Source: CAD feature listing. Evaluate the final solid. Frame: model axes, mm. A direction names the side the tool comes from. Round coordinates to 2 decimals unless told otherwise and drop trailing zeros. Loops run counter-clockwise (first coordinate to the right, second up) from the corner with the lowest first, then second, coordinate; pieces in that order, holes last. Notation, with made-up numbers: M 66.5,30.5 L 89.5,30.5 A13 cw 89.5,44.5 Z; hole C -25,0 d10. An arc over 180 degrees is marked long. Answer as CSV lines item,"result". Start each with the question number.
Autodesk Fusion 360 part; units mm, degrees
sketch "Sketch1" plane through (0, 0, 0) normal (0, 0, 1) x (1, 0, 0)
  line L0 (9, 9) -> (-9, 9) construction
  line L1 (-9, 9) -> (-9, -9) construction
  line L2 (-9, -9) -> (9, -9) construction
  line L3 (9, -9) -> (9, 9) construction
  line L4 (9, 9) -> (-9, -9) construction
  line L5 (-9, 9) -> (9, -9) construction
  line L6 (-6.4, 8) -> (6.4, 8)
  line L7 (6.4, 8) -> (6.4, -5.4)
  line L8 (6.4, -5.4) -> (-6.4, -5.4)
  line L9 (-6.4, -5.4) -> (-6.4, 8)
  circle A0 centre (0, 0) radius 3.5
  line L10 (2.4, -0.6) -> (-2.4, -0.6)
  line L11 (-2.4, -0.6) -> (-2.4, 0.6)
  line L12 (-2.4, 0.6) -> (2.4, 0.6)
  line L13 (2.4, 0.6) -> (2.4, -0.6)
  line L14 (2.4, -0.6) -> (-2.4, 0.6) construction
  line L15 (-2.4, -0.6) -> (2.4, 0.6) construction
  line L16 (0.6, -2.4) -> (-0.6, -2.4)
  line L17 (-0.6, -2.4) -> (-0.6, 2.4)
  line L18 (-0.6, 2.4) -> (0.6, 2.4)
  line L19 (0.6, 2.4) -> (0.6, -2.4)
  line L20 (0.6, -2.4) -> (-0.6, 2.4) construction
  line L21 (-0.6, -2.4) -> (0.6, 2.4) construction
  line L22 (-0.6, 2.4) -> (-2.5475, 2.4)
  line L23 (0.6, 2.4) -> (2.5475, 2.4)
  line L24 (-0.6, -2.4) -> (-2.5475, -2.4)
  line L25 (0.6, -2.4) -> (2.5475, -2.4)
  dimension "d1" = 18
  dimension "d2" = 18
  dimension "d3" = 3.6
  dimension "d4" = 1
  dimension "d5" = 2.6
  dimension "d6" = 2.6
  dimension "d7" = 7
  dimension "d8" = 4.8
  dimension "d9" = 1.2
  dimension "d10" = 1.2
  dimension "d11" = 4.8
extrude "Extrude1" add sketch "Sketch1" along normal blind 0.6 contours L6 L7 L8 L9 | A0 L10 L12 L13 L19 L23 L25 | A0 L18 L22 L23 | A0 L16 L24 L25 | A0 L10 L11 L12 L17 L22 L24 | L12 L17 L18 L19 | L10 L16 L17 L19 | L10 L12 L17 L19 | L10 L12 L13 L19 | L10 L11 L12 L17
extrude "Extrude2" add sketch "Sketch1" along normal blind 4 contours A0 L10 L12 L13 L19 L23 L25 | A0 L10 L11 L12 L17 L22 L24
fillet "Fillet1" radius 1 6 edges at (-1.5738, -2.4, 0.6) (-3.5, 0, 0.6) (1.5738, -2.4, 0.6) (3.5, 0, 0.6) (1.5738, 2.4, 0.6) (-1.5738, 2.4, 0.6)
fillet "Fillet1" radius 0.5 4 edges at (6.4, 8, 0.3) (-6.4, 8, 0.3) (6.4, -5.4, 0.3) (-6.4, -5.4, 0.3)
chamfer "Chamfer1" distance 0.4 angle 45 20 edges at (-6.2536, 7.8536, 0) (0, 8, 0) (6.2536, 7.8536, 0) (6.4, 1.3, 0) (6.2536, -5.2536, 0) (0, -5.4, 0) (-6.2536, -5.2536, 0) (-6.4, 1.3, 0) (-0.6, 1.5, 4) (-1.5, 0.6, 4) (-2.4, 0, 4) (-1.5, -0.6, 4) (-0.6, -1.5, 4) (0.6, -1.5, 4) (1.5, -0.6, 4) (2.4, 0, 4) (1.5, 0.6, 4) (0.6, 1.5, 4) (3.5, 0, 4) (-3.5, 0, 4)
1) Section C-C, the plane y = 3.75. Return loops of the section in (x, z).
2) Ray query, line 1 along X through (y, z) = (0, 2.9); line 2 along Y through (x, z) = (0.75, 3.5); line 3 along Z through (x, y) = (-2.25, -3.5). Return the intervals inside material, ascending.
3) Section D-D, the plane x = 5.5. Return loops of the section in (y, z), and give its area (3 significant figures).
4) Contact query for flat-ended pins moving along their axis: pin 1 Ø0.8 at (y, z) = (-2, 2.5) entering from -X; pin 2 Ø2 at (x, z) = (1.5, 2.5) entering from -Y (3 decimals); pin 3 Ø2 at (x, z) = (1.5, 3) entering from +Y. Output: stop coordinate, or through.
5) Access query for faces 1 (the flat face through (-2.4, 0, 2)), 2 (the flat face through (-0.6, 2, 2)), 3 (the flat face through (2, 2.4, 3)). Directions: +Z, -Z, +X, -X, +Y, -Y. A direction counts if a zero-diameter tool reaches every point of the face in a straight line with its end or side. Return the directions, or none.
6) Mould query, pull axis X, two halves, no side actions, for faces 4 (the flat face through (0, 1, 0)), 5 (the conical face through (3.21, 0.04, 3.89)), 6 (the flat face through (1, 0.6, 2)). Classes: pulls with the +X half, pulls with the -X half, needs draft (parallel to the pull), parting line crosses it, or undercut.
7) Section A-A, the plane x = -1.5. Return loops of the section in (y, z), and give its area (3 significant figures).
8) Section B-B, the plane z = 2.35. Return loops of the section in (x, y), and give its area (3 significant figures).
Findings below:
1,outline,"M -6.4,0.4 L -6,0 L 6,0 L 6.4,0.4 L 6.4,0.6 L -6.4,0.6 Z"
2,line 1,"-3.5 to -2.4, 2.4 to 3.5"
2,line 2,"-2.4 to -0.6, 0.6 to 2.4"
2,line 3,"0 to 0.6"
3,outline,"M -5.4,0.4 L -5,0 L 7.6,0 L 8,0.4 L 8,0.6 L -5.4,0.6 Z"
3,area,"7.88 mm²"
4,pin 1,"x = -3.11"
4,pin 2,"y = -2.405"
4,pin 3,"y = 2.4"
5,face 1,"+Z"
5,face 2,"+Z, +Y, -Y"
5,face 3,"+Z, +X, -X, +Y"
6,face 4,"needs draft"
6,face 5,"pulls with the +X half"
6,face 6,"undercut"
7,outline,"M -5.4,0.4 L -5,0 L 7.6,0 L 8,0.4 L 8,0.6 L 3.4,0.6 A1 cw 2.4,1.6 L 2.4,4 L 1,4 L 0.6,3.6 L 0.6,0.6 L -0.6,0.6 L -0.6,3.6 L -1,4 L -2.4,4 L -2.4,1.6 A1 cw -3.4,0.6 L -5.4,0.6 Z"
7,area,"20.4 mm²"
8,outline,"M -2.55,-2.4 L -0.6,-2.4 L -0.6,-0.6 L -2.4,-0.6 L -2.4,0.6 L -0.6,0.6 L -0.6,2.4 L -2.55,2.4 A3.5 ccw Z; M 0.6,-2.4 L 2.55,-2.4 A3.5 ccw 2.55,2.4 L 0.6,2.4 L 0.6,0.6 L 2.4,0.6 L 2.4,-0.6 L 0.6,-0.6 Z"
8,area,"20.7 mm²"
